Read the model definition and answer for the solid it produces. Units are mm, in the model's axes. Round coordinates to 2 decimals unless told otherwise and drop trailing zeros. Order: outer loops, then holes, each group sorted by start corner. A loop starts at its lowest first (then second) coordinate and runs counter-clockwise, first axis right, second up. Notation, with made-up numbers: (69, 64) - (115, 64) arc R20 ccw to (115, 79) - close; hole circle Ø4 at (-26, 35.25). An arc over 180 degrees is marked (long way). Put each result on its own line as item: value. Start each with the question number.
Q1. Section B-B on z = -36.5 is taken. Give the vertices of the cut face in (x, y).
Q2. For a pull along X with two mould halves and no side action, classify faces 1 (the face through (-11.056, 550.977, 49.787)), 2 (the face through (-11.084, 550.977, 48.372)), 3 (the face through (49, 0, 7)) as pulls with the +X half, pulls with the -X half, needs draft (parallel to the pull), parting line crosses it, or undercut.
Q3. Find the intervals of material crossed by line 1 along X through (y, z) = (472, 0); line 2 along Z through (x, y) = (-3, 813.5); line 3 along Z through (x, y) = (-4, 877.5), in increasing order. Write a range as from..to.
Q4. Section A-A on x = 27 is taken. Give the vertices of the cut face in (y, z).
Q5. Each of these flat-tipped pins is pushed along its axis until it touches: pin 1 Ø1.5 at (x, y) = (39.5, 344.5) entering from -Z; pin 2 Ø1 at (x, y) = (-25.5, 905) entering from +Z; pin 3 Ø1 at (y, z) = (856, -18) entering from -X. Where does it stop, or does it pass through?
Q6. Section C-C on y = 569 is taken. Give the vertices of the cut face in (x, z), then the cut area to 3 significant figures.
from build123d import *

# Parameters (mm, degrees)
SKETCH1_R           = 51
SKETCH1_R_2         = 49.55
BOSS_EXTRUDE1_DEPTH = 1117.6
CUT_EXTRUDE1_DEPTH  = 52
CIRPATTERN1_COUNT   = 3


with BuildPart() as part:
    # Sketch1 → Boss-Extrude1 (new body)
    with BuildSketch(Plane(origin=(0, 0, 0), x_dir=(1, 0, 0), z_dir=(0, 1, 0))):
        Circle(SKETCH1_R)
        with Locations((-0.342312985, 0)):
            Circle(SKETCH1_R_2, mode=Mode.SUBTRACT)
    extrude(amount=BOSS_EXTRUDE1_DEPTH)

    # Sketch2 → Cut-Extrude1 (cut, through all)
    with BuildSketch(Plane.XY):
        Polygon((0, 12.7), (2.38, 12.7), (2.38, 383.7), (-2.38, 383.7), (-2.38, 12.7), align=None)
    cut_extrude1 = extrude(amount=-CUT_EXTRUDE1_DEPTH, mode=Mode.SUBTRACT)

    # CirPattern1: Cut-Extrude1 ×3 about axis
    cirpattern1_axis = Axis((0, 0, 0), (0, 1, 0))
    for i in range(1, CIRPATTERN1_COUNT):
        add(cut_extrude1.rotate(cirpattern1_axis, i * 360 / CIRPATTERN1_COUNT), mode=Mode.SUBTRACT)


solid = part.part
Findings:
1. outline: (-35.62, 0) - (-33.85, 0) - (-33.85, 1117.6) - (-35.62, 1117.6) - close; (33.17, 0) - (35.62, 0) - (35.62, 1117.6) - (33.17, 1117.6) - close
2. face 1: parting line crosses it
2. face 2: undercut
2. face 3: needs draft
3. line 1: -51..-49.89, 49.21..51
3. line 2: -50.91..-49.48, 49.48..50.91
3. line 3: -50.84..-49.41, 49.41..50.84
4. outline: (0, -43.27) - (1117.6, -43.27) - (1117.6, -41.32) - (0, -41.32) - close; (0, 41.32) - (1117.6, 41.32) - (1117.6, 43.27) - (0, 43.27) - close
5. pin 1: z = -33.16
5. pin 2: z = 44.45
5. pin 3: x = -47.9
6. outline: circle Ø102 at (0, 0); hole circle Ø99.1 at (-0.34, 0)
6. area: 458 mm2
